CAD build for the part. Positions are in the model's coordinates, mm. Give positions to 0.01 mm unless a question says otherwise; leave off trailing zeros. Write each loop counter-clockwise with the first axis right and the second up, starting at its lowest first coordinate (ties: lowest second). Pieces come first, ordered by that corner, then holes. Notation, with made-up numbers: (45, 47.25) - (66, 47.25) arc R27 cw to (66, 65.25) - close; hole circle Ø7 at (-23, 0.25). An arc over 180 degrees is marked (long way). Answer as a JSON object with one key per item and string values.
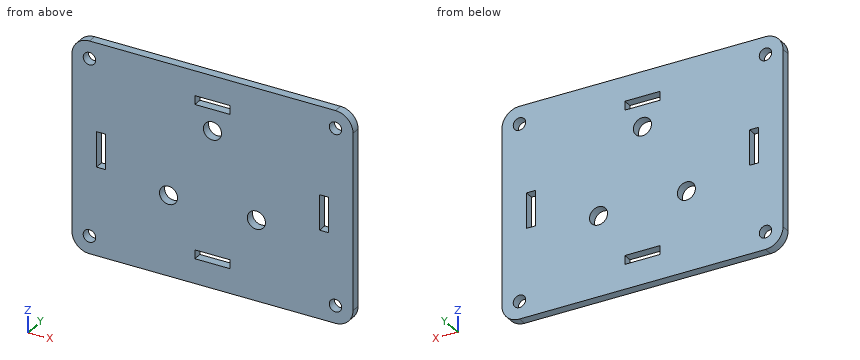
from build123d import *

# Parameters (mm, degrees)
SKETCH1_W           = 101.6
SKETCH1_H           = 76.2
BOSS_EXTRUDE1_DEPTH = 3.175
FILLET1_R           = 6.35
SKETCH2_R           = 2.2479
CUT_EXTRUDE1_DEPTH  = 4.175
SKETCH3_R           = 3.2639
CUT_EXTRUDE2_DEPTH  = 4.175


with BuildPart() as part:
    # Sketch1 → Boss-Extrude1 (new body)
    with BuildSketch(Plane(origin=(0, 0, 0), x_dir=(1, 0, 0), z_dir=(0, 1, 0))):
        Rectangle(SKETCH1_W, SKETCH1_H)
    extrude(amount=BOSS_EXTRUDE1_DEPTH)

    # Fillet1
    fillet1_edges = [part.edges().sort_by_distance(p)[0] for p in [
        (50.8, 1.5875, 38.1),
        (-50.8, 1.5875, 38.1),
        (-50.8, 1.5875, -38.1),
        (50.8, 1.5875, -38.1),
    ]]
    fillet(fillet1_edges, radius=FILLET1_R)

    # Sketch2 → Cut-Extrude1 (cut, through all)
    with BuildSketch(Plane(origin=(0, 3.175, 0), x_dir=(1, 0, 0), z_dir=(0, 1, 0))):
        with Locations((-44.45, 31.75)):
            Circle(SKETCH2_R)
        with Locations((44.45, 31.75)):
            Circle(SKETCH2_R)
        with Locations((44.45, -31.75)):
            Circle(SKETCH2_R)
        with Locations((-44.45, -31.75)):
            Circle(SKETCH2_R)
        Polygon((-41.91, 0), (-41.91, 6.35), (-38.735, 6.35), (-38.735, -6.35), (-41.91, -6.35), align=None)
        Polygon((0, 29.21), (6.35, 29.21), (6.35, 26.035), (-6.35, 26.035), (-6.35, 29.21), align=None)
        Polygon((41.91, 0), (41.91, 6.35), (38.735, 6.35), (38.735, -6.35), (41.91, -6.35), align=None)
        Polygon((0, -29.21), (6.35, -29.21), (6.35, -26.035), (-6.35, -26.035), (-6.35, -29.21), align=None)
    extrude(amount=-CUT_EXTRUDE1_DEPTH, mode=Mode.SUBTRACT)

    # Sketch3 → Cut-Extrude2 (cut, through all)
    with BuildSketch(Plane(origin=(0, 3.175, 0), x_dir=(1, 0, 0), z_dir=(0, 1, 0))):
        with Locations((-15.875, 9.165435523)):
            Circle(SKETCH3_R)
        with Locations((15.875, 9.165435523)):
            Circle(SKETCH3_R)
        with Locations((0, -18.330871047)):
            Circle(SKETCH3_R)
    extrude(amount=-CUT_EXTRUDE2_DEPTH, mode=Mode.SUBTRACT)


solid = part.part
(1) Saw through at A-A, the plane z = 1. Give the cut face in (x, y) (3 decimals).
Answer key:
{"outline": "(-50.8, 0) - (-41.91, 0) - (-41.91, 3.175) - (-50.8, 3.175) - close; (-38.735, 0) - (38.735, 0) - (38.735, 3.175) - (-38.735, 3.175) - close; (41.91, 0) - (50.8, 0) - (50.8, 3.175) - (41.91, 3.175) - close"}
(2) Saw through at B-B, the plane z = 27.5. Give the cut face in (x, y) (3 decimals), and give its area (3 significant figures).
Answer key:
{"outline": "(-50.8, 0) - (-6.35, 0) - (-6.35, 3.175) - (-50.8, 3.175) - close; (6.35, 0) - (50.8, 0) - (50.8, 3.175) - (6.35, 3.175) - close", "area": "282 mm²"}
(3) Saw through at D-D, the plane y = 0.7. State how many separate pieces and enclosed holes the cut face has, and give its area (3 significant figures).
Answer key:
{"separate pieces": "1", "enclosed holes": "11", "area": "7,380 mm²"}
(4) Saw through at C-C, the plane x = 0. Give the cut face in (y, z) (3 decimals).
Answer key:
{"outline": "(0, -38.1) - (3.175, -38.1) - (3.175, -29.21) - (0, -29.21) - close; (0, -26.035) - (3.175, -26.035) - (3.175, 15.067) - (0, 15.067) - close; (0, 21.595) - (3.175, 21.595) - (3.175, 26.035) - (0, 26.035) - close; (0, 29.21) - (3.175, 29.21) - (3.175, 38.1) - (0, 38.1) - close"}
(5) Probe L1, parallel to Z at x = 44.45, y = 1.85; L2, parallel to X at y = 1.85, z = -31.5; L3, parallel to X at y = 0.3, z = 1.5 (3 decimals). List the from-to ranges inside material, lowest first. Write a range as [from, to].
Answer key:
{"L1": "z = [-38.1, -34], [-29.5, 29.5], [34, 38.1]", "L2": "x = [-50.8, -46.68], [-42.22, 42.22], [46.68, 50.8]", "L3": "x = [-50.8, -41.91], [-38.735, 38.735], [41.91, 50.8]"}
